Source: three-view drawing plus pictorial views. Frame: mm from the lowest corner of the part. Coordinates: 2 decimals unless noted, no trailing zeros. Write each loop counter-clockwise with the first axis right and the second up, starting at its lowest first coordinate (ties: lowest second). Pieces come first, ordered by that corner, then holes. Notation, with made-up numbers: (24.5, 22) -> (79.5, 22) arc R21 cw to (79.5, 46) -> close; hole circle Ø10 at (57.25, 73.5). An arc over 180 degrees is marked (long way). One line per question, with ' | ' between items. Start each with the question number.
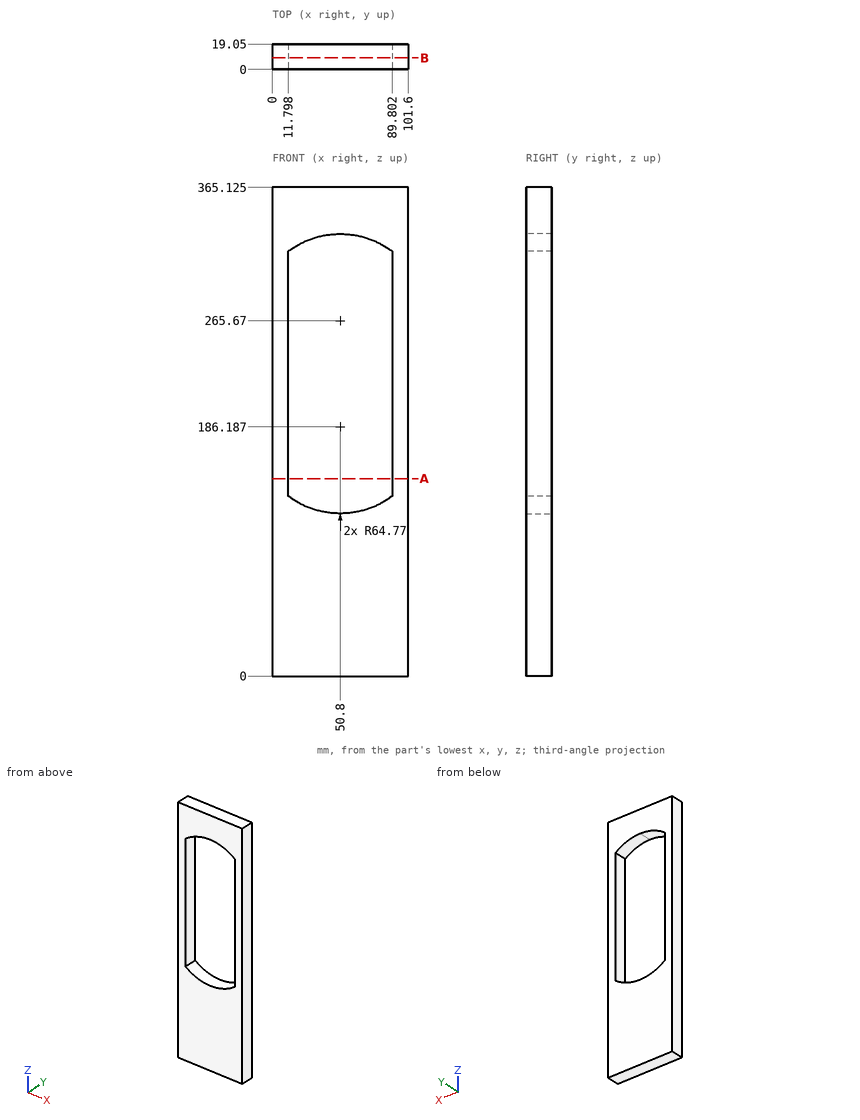
1) Section A-A, the plane z = 147.5. Return loops of the section in (x, y).
2) Ray query, line 1 (X direction, y = 3, z = 253); line 2 (Z direction, x = 49, y = 7.75) (1 decimal); line 3 (Z direction, x = 34, y = 7.5) (1 decimal). Return the intervals inside material, ascending.
3) Section B-B, the plane y = 8.75. Return loops of the section in (x, z) (1 decimal), then the cut area to 3 significant figures.
Answer block:
1) outline: (0, 0) -> (11.8, 0) -> (11.8, 19.05) -> (0, 19.05) -> close; (89.8, 0) -> (101.6, 0) -> (101.6, 19.05) -> (89.8, 19.05) -> close
2) line 1: x = 0 to 11.8, 89.8 to 101.6 | line 2: z = 0 to 121.4, 330.4 to 365.1 | line 3: z = 0 to 123.6, 328.2 to 365.1
3) outline: (0, 0) -> (101.6, 0) -> (101.6, 365.1) -> (0, 365.1) -> close; hole (11.8, 134.5) arc R64.8 ccw to (89.8, 134.5) -> (89.8, 317.4) arc R64.8 ccw to (50.8, 330.4) arc R64.8 ccw to (11.8, 317.4) -> close | area: 21,400 mm2
